Read the model definition and answer for the solid it produces. Units are mm, in the model's axes. Face numbers are marked on the shaded views. Round coordinates to 2 decimals unless told otherwise and drop trailing zeros. Order: outer loops, then holes, each group sorted by start corner. A loop starts at its lowest first (then second) coordinate and runs counter-clockwise, first axis right, second up. Notation, with made-up numbers: (21, 23.25) - (25, 23.25) arc R11 cw to (25, 43.25) - close; hole circle Ø11 at (8.25, 48.5). An arc over 180 degrees is marked (long way). Put each result on its own line as item: value. Start each with the question number.
Q1. Find the intervals of material crossed by line 1 along Z through (x, y) = (32, 2.2); line 2 along X through (y, z) = (0.45, 42.5); line 3 along Z through (x, y) = (56, 2.9), in increasing order. Write a range as from..to.
Q2. For a pull along Z with two mould halves and no side action, classify the marked faces 1 and 2 as pulls with the +Z half, pulls with the -Z half, needs draft (parallel to the pull), parting line crosses it, or undercut.
Q3. Section A-A on y = 2.9 is taken. Give the vertices of the cut face in (x, z), then the cut area to 3 significant figures.
Q4. Section B-B on x = -8.5 is taken. Give the vertices of the cut face in (y, z), then the cut area to 3 significant figures.
Q5. Section C-C on z = 19.5 is taken. Give the vertices of the cut face in (x, y), then the cut area to 4 significant figures.
Q6. Section D-D on x = 18.5 is taken. Give the vertices of the cut face in (y, z), then the cut area to 3 significant figures.
Q7. Each of these flat-tipped pins is pushed along its axis until it touches: pin 1 Ø1.5 at (x, z) = (30.5, 17) entering from +Y; pin 2 Ø1.6 at (y, z) = (3, 43.5) entering from +X; pin 3 Ø0.6 at (x, y) = (27, 2.5) entering from +Z. Where does it stop, or does it pass through?
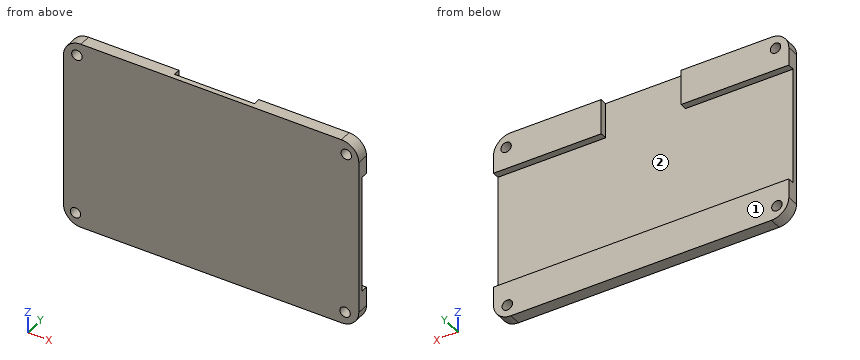
from build123d import *

# Parameters (mm, degrees)
BOSS_EXTRUDE1_DEPTH = 3.5
SKETCH2_R           = 1.5
CUT_EXTRUDE1_DEPTH  = 3.5
SKETCH3_W           = 23
SKETCH3_H           = 10.283770076
CUT_EXTRUDE2_DEPTH  = 2


with BuildPart() as part:
    # Sketch1 → Boss-Extrude1 (new body)
    with BuildSketch(Plane(origin=(0, 0, 0), x_dir=(1, 0, 0), z_dir=(0, 1, 0))):
        with BuildLine():
            Line((-20.62248996, 7.565261044), (54.37751004, 7.565261044))
            ThreePointArc((54.37751004, 7.565261044), (57.913043946, 6.10079495), (59.37751004, 2.565261044))
            Line((59.37751004, 2.565261044), (59.37751004, -42.434738956))
            ThreePointArc((59.37751004, -42.434738956), (57.913043946, -45.970272862), (54.37751004, -47.434738956))
            Line((54.37751004, -47.434738956), (-20.62248996, -47.434738956))
            ThreePointArc((-20.62248996, -47.434738956), (-24.158023866, -45.970272862), (-25.62248996, -42.434738956))
            Line((-25.62248996, -42.434738956), (-25.62248996, 2.565261044))
            ThreePointArc((-25.62248996, 2.565261044), (-24.158023866, 6.10079495), (-20.62248996, 7.565261044))
        make_face()
    extrude(amount=BOSS_EXTRUDE1_DEPTH)

    # Sketch2 → Cut-Extrude1 (cut)
    with BuildSketch(Plane(origin=(0, 3.5, 0), x_dir=(1, 0, 0), z_dir=(0, 1, 0))):
        with Locations((-22.187566987, 3.802718615)):
            Circle(SKETCH2_R)
        with Locations((55.412433013, 3.947865339)):
            Circle(SKETCH2_R)
        with Locations((55.766505812, -43.552134661)):
            Circle(SKETCH2_R)
        with Locations((-21.775437199, -43.697281385)):
            Circle(SKETCH2_R)
    extrude(amount=-CUT_EXTRUDE1_DEPTH, mode=Mode.SUBTRACT)

    # Sketch3 → Cut-Extrude2 (cut)
    with BuildSketch(Plane(origin=(0, 3.5, 0), x_dir=(1, 0, 0), z_dir=(0, 1, 0))):
        with Locations((16.87751004, -42.292853918)):
            Rectangle(SKETCH3_W, SKETCH3_H)
        Polygon((59.37751004, -2.947281385), (-25.62248996, -2.947281385), (-25.62248996, -37.15096888), (5.37751004, -37.15096888), (28.37751004, -37.15096888), (59.37751004, -37.15096888), align=None)
    extrude(amount=-CUT_EXTRUDE2_DEPTH, mode=Mode.SUBTRACT)


solid = part.part
Findings:
1. line 1: -7.57..2.95, 37.15..47.43
1. line 2: -25.62..-22.68, -20.87..54.7, 56.84..59.38
1. line 3: -7.29..-5.33, -2.57..2.95, 37.15..42.07, 45.03..47.16
2. face 1: needs draft
2. face 2: undercut
3. outline: (-25.62, -2.57) arc R5 ccw to (-20.62, -7.57) - (54.38, -7.57) arc R5 ccw to (59.38, -2.57) - (59.38, 2.95) - (-25.62, 2.95) - close; (-25.62, 37.15) - (5.38, 37.15) - (5.38, 47.43) - (-20.62, 47.43) arc R5 ccw to (-25.62, 42.43) - close; (28.38, 37.15) - (59.38, 37.15) - (59.38, 42.43) arc R5 ccw to (54.38, 47.43) - (28.38, 47.43) - close; hole circle Ø3 at (-22.19, -3.8); hole circle Ø3 at (-21.78, 43.7); hole circle Ø3 at (55.41, -3.95); hole circle Ø3 at (55.77, 43.55)
3. area: 1,480 mm2
4. outline: (0, -7.57) - (3.5, -7.57) - (3.5, 2.95) - (1.5, 2.95) - (1.5, 37.15) - (3.5, 37.15) - (3.5, 47.43) - (0, 47.43) - close
4. area: 124 mm2
5. outline: (-25.62, 0) - (59.38, 0) - (59.38, 1.5) - (-25.62, 1.5) - close
5. area: 127.5 mm2
6. outline: (0, -7.57) - (3.5, -7.57) - (3.5, 2.95) - (1.5, 2.95) - (1.5, 47.43) - (0, 47.43) - close
6. area: 104 mm2
7. pin 1: y = 1.5
7. pin 2: x = 59.37
7. pin 3: z = 2.95
